Model file for the job. Use its own axes, mm. A direction names the side the tool comes from. Give positions to 0.01 mm unless a question says otherwise; leave off trailing zeros. Write each loop counter-clockwise with the first axis right and the second up, starting at its lowest first coordinate (ties: lowest second). Pieces come first, ordered by that corner, then holes.
Autodesk Inventor part; units mm, degrees
ref_plane "YZ Plane" through (0, 0, 0) normal (1, 0, 0) x (0, 1, 0)
ref_plane "XZ Plane" through (0, 0, 0) normal (0, 1, 0) x (-1, 0, 0)
ref_plane "XY Plane" through (0, 0, 0) normal (0, 0, 1) x (1, 0, 0)
sketch "スケッチ1" plane through (0, 0, 0) normal (0, 0, 1) x (1, 0, 0)
  line L0 (-30.25, 12.5) -> (30.25, 12.5)
  line L1 (30.25, 12.5) -> (30.25, -12.5)
  line L2 (30.25, -12.5) -> (-30.25, -12.5)
  line L3 (-30.25, -12.5) -> (-30.25, 12.5)
  line L4 (-25.25, 9.5) -> (25.25, 9.5) construction
  line L5 (25.25, 9.5) -> (25.25, -9.5) construction
  line L6 (25.25, -9.5) -> (-25.25, -9.5) construction
  line L7 (-25.25, -9.5) -> (-25.25, 9.5) construction
  line L8 (25.25, 9.5) -> (-25.25, -9.5) construction
  line L9 (-25.25, -7.8973) -> (-25.25, 9.5)
  line L10 (-25.25, 9.5) -> (20.9903, 9.5)
  line L11 (20.9903, 9.5) -> (-25.25, -7.8973)
  line L12 (-20.9903, -9.5) -> (25.25, -9.5)
  line L13 (25.25, -9.5) -> (25.25, 7.8973)
  line L14 (25.25, 7.8973) -> (-20.9903, -9.5)
  line L15 (-30.25, 10) -> (30.25, 10) construction
  line L16 (30.25, -10) -> (-30.25, -10) construction
  line L17 (30.25, 10) -> (30.25, -10) construction
  point P0 (0, 0)
  point P1 (0, 9.5)
  point P2 (0, 12.5)
  point P3 (25.25, 0)
  point P4 (30.25, 0)
  dimension "d0" = 5
  dimension "d1" = 3
  dimension "d2" = 1.5
  dimension "d4" = 2.5
  dimension "d16" = 60.5
  dimension "d17" = 25
  dimension "d18" = 20
extrude "押し出し1" add sketch "スケッチ1" along normal blind 5
sketch "スケッチ2" plane through (30.25, -12.5, 0) normal (1, 0, 0) x (0, 0, -1)
  line L0 (0, 25) -> (-5, 25)
  line L1 (-5, 0) -> (-5, 25)
  line L2 (0, 12.5) -> (-5, 12.5) construction
  point P0 (-2.5, 2.5)
  point P1 (-2.5, 22.5)
  point P2 (-2.5, 25)
  dimension "d7" = 20
hole "穴1" at (30.25, -10, 2.5) at (30.25, 10, 2.5) direction (-1, 0, 0) diameter 2.459 depth 3
mirror "ミラー1" about plane through (0, 0, 0) normal (1, 0, 0) of "穴1"
fillet "フィレット1" radius 2 6 edges at (-20.9903, -9.5, 2.5) (-25.25, -7.8973, 2.5) (25.25, 7.8973, 2.5) (25.25, -9.5, 2.5) (-25.25, 9.5, 2.5) (20.9903, 9.5, 2.5)
equation "\"d3\" = d5_1"
equation "\"d5_1\" = 24"
properties part number "BackLink_diagonal" material "アルミニウム 2014-T4"
1. Slice it at D-D, the plane x = -21.5. Write the cut outline in (y, z), and give its area (3 significant figures).
Calculated:
outline: (-12.5, 0) - (-6.49, 0) - (-6.49, 5) - (-12.5, 5) - close; (9.5, 0) - (12.5, 0) - (12.5, 5) - (9.5, 5) - close
area: 45.1 mm2
2. Slice it at C-C, the plane y = -1.5. Write the cut outline in (x, z), and give its area (3 significant figures).
Calculated:
outline: (-30.25, 0) - (-25.25, 0) - (-25.25, 5) - (-30.25, 5) - close; (-8.25, 0) - (0.27, 0) - (0.27, 5) - (-8.25, 5) - close; (25.25, 0) - (30.25, 0) - (30.25, 5) - (25.25, 5) - close
area: 92.6 mm2
3. Pin check, flat tips, straight feed: P1, Ø1.2, axis at y = -9.5, z = 2, coming from the +X side; P2, Ø0.7, axis at y = 9.5, z = 2.5, coming from the +X side; P3, Ø1.5, axis at y = 10, z = 2.5, coming from the -X side; P4, Ø4, axis at x = 2, y = -4.5, coming from the -Z side. Stop position of each tip, or through.
Calculated:
P1: stops at x = 30.25
P2: stops at x = 27.25
P3: stops at x = -27.25
P4: passes through
4. Slice it at A-A, the plane z = 2.5. State how many separate pieces and enclosed holes the cut face has, and give its area (3 significant figures).
Calculated:
separate pieces: 1
enclosed holes: 2
area: 717 mm2
5. Slice it at B-B, the plane x = 19.5. Write the cut outline in (y, z), and give its area (3 significant figures).
Calculated:
outline: (-12.5, 0) - (-9.5, 0) - (-9.5, 5) - (-12.5, 5) - close; (5.73, 0) - (12.5, 0) - (12.5, 5) - (5.73, 5) - close
area: 48.8 mm2
6. Pull direction Y, two halves, no side cores. Call faces 5 (the flat face through (0, 0, 0)), 6 (the flat face through (0, -12.5, 2)), 7 (the flat face through (27.25, -10, 3)): +Y half, -Y half, draft (parallel to the pull), parting line (faces both ways), or undercut.
Calculated:
face 5: draft
face 6: -Y half
face 7: undercut
7. Which spindle directions (+Z, -Z, +X, -X, +Y, -Y) get a long thin tool onto all of the face, cutting with end or side? Do faces 1 (the flat face through (0, 0, 5)), 2 (the cylindrical face through (28.729, -10.369, 1.327)), 3 (the cylindrical face through (-28.73, -11.09, 1.93)), 4 (the cylindrical face through (24.41, 6.637, 2.535)). Say none if no direction does.
Calculated:
face 1: +Z, +X, -X, +Y, -Y
face 2: +X
face 3: -X
face 4: +Z, -Z
8. Probe probe 1 along Y at (x, z) = (29.6, 2.5); probe 2 along Z at (x, y) = (27.9, 10); probe 3 along Y at (x, z) = (-7.5, 2.7). List the from-to ranges inside material, lowest first.
Calculated:
probe 1: y = -12.5 to -11.23, -8.77 to 8.77, 11.23 to 12.5
probe 2: z = 0 to 1.27, 3.73 to 5
probe 3: y = -12.5 to -9.5, -4.42 to -1.22, 9.5 to 12.5
